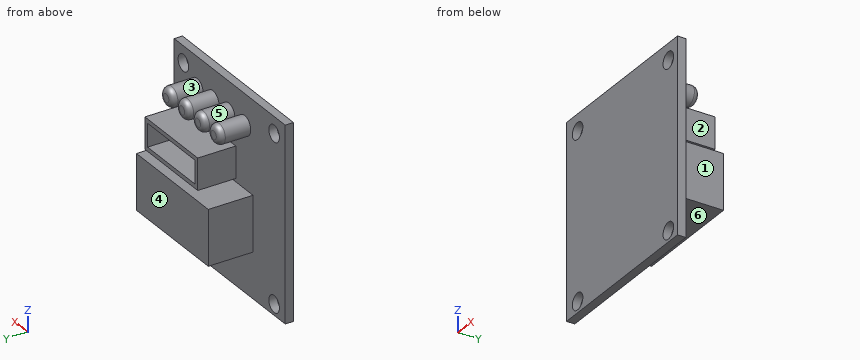
Autodesk Inventor part; units mm, degrees
ref_plane "YZ Plane" through (0, 0, 0) normal (1, 0, 0) x (0, 1, 0)
ref_plane "XZ Plane" through (0, 0, 0) normal (0, 1, 0) x (-1, 0, 0)
ref_plane "XY Plane" through (0, 0, 0) normal (0, 0, 1) x (1, 0, 0)
sketch "Sketch1" plane through (0, 0, 0) normal (0, 1, 0) x (-1, 0, 0)
  line L0 (0, 0) -> (-31.55, 0)
  line L1 (-31.55, 0) -> (-31.55, -35)
  line L2 (-31.55, -35) -> (0, -35)
  line L3 (0, -35) -> (0, 0)
  circle A0 centre (-3.15, -33) radius 1.5
  circle A1 centre (-28.95, -33) radius 1.5
  circle A2 centre (-3.15, -3) radius 1.5
  circle A3 centre (-28.95, -3) radius 1.5
  dimension "d0" = 31.55
  dimension "d1" = 35
  dimension "d2" = 3
  dimension "d3" = 25.8
  dimension "d4" = 2.6
  dimension "d5" = 30
  dimension "d6" = 2
extrude "Extrusion1" add sketch "Sketch1" along normal blind 1.5
sketch "Sketch2" plane through (0, 1.5, 0) normal (0, 1, 0) x (1, 0, 0)
  line L0 (9.15, 26.76) -> (29.55, 26.76)
  line L1 (29.55, 26.76) -> (29.55, 16.76)
  line L2 (29.55, 16.76) -> (9.15, 16.76)
  line L3 (9.15, 16.76) -> (9.15, 26.76)
  line L4 (31.55, 35) -> (0, 35)
  line L5 (29.05, 16.16) -> (14.05, 16.16)
  line L6 (14.05, 16.16) -> (14.05, 10.45)
  line L7 (14.05, 10.45) -> (29.05, 10.45)
  line L8 (29.05, 10.45) -> (29.05, 16.16)
  line L9 (28.3, 11.2) -> (14.8, 11.2)
  line L10 (14.8, 11.2) -> (14.8, 15.41)
  line L11 (14.8, 15.41) -> (28.3, 15.41)
  line L12 (28.3, 15.41) -> (28.3, 11.2)
  line L13 (31.55, 0) -> (31.55, 35)
  circle A0 centre (11.55, 5.6) radius 1.75
  circle A1 centre (16.05, 5.6) radius 1.75
  circle A2 centre (20.55, 5.6) radius 1.75
  circle A3 centre (25.05, 5.6) radius 1.75
  line L14 (0, 0) -> (31.55, 0)
  dimension "d9" = 10
  dimension "d10" = 20.4
  dimension "d11" = 8.24
  dimension "d12" = 2
  dimension "d15" = 15
  dimension "d16" = 5.71
  dimension "d17" = 2.5
  dimension "d18" = 10.45
  dimension "d19" = 0.75
  dimension "d22" = 4.5
  dimension "d23" = 4.5
  dimension "d24" = 4.5
  dimension "d25" = 6.5
  dimension "d26" = 5.6
  dimension "d27" = 3.5
extrude "Extrusion2" add sketch "Sketch2" along normal blind 8.11 contours L0 L1 L2 L3
extrude "Extrusion3" add sketch "Sketch2" along normal blind 6.9 contours L8 L7 L6 L5
extrude "Extrusion4" add sketch "Sketch2" along normal blind 5.6 contours A0 | A1 | A2 | A3
fillet "Fillet1" radius 1 4 edges at (9.8, 7.1, -5.6) (14.3, 7.1, -5.6) (18.8, 7.1, -5.6) (23.3, 7.1, -5.6)
properties part number "STEPPER DRIVER"
Design review of the part built by this model. Coordinates are the model's own, in mm. Face numbers are marked on the shaded views. A direction names the side the tool comes from. Give positions to 0.01 mm unless a question says otherwise; leave off trailing zeros. Order: outer loops, then holes, each group sorted by start corner. A loop starts at its lowest first (then second) coordinate and runs counter-clockwise, first axis right, second up. Notation, with made-up numbers: (40.25, -5.5) - (64.25, -5.5) arc R35 cw to (64.25, 33.5) - close; hole circle Ø4 at (77.5, 13.5). An arc over 180 degrees is marked (long way). Use CSV: the item, a comma, the result in double quotes. Start each with the question number.
Q1. Machinability: for the marked faces 1, 2 and 3, which of the approach directions +Z, -Z, +X, -X, +Y, -Y give a long, thin tool a straight path to every point of the face, cutting with its end or side? Answer none if there is none.
Q2. Take a section at D-D (z = -13). State the section outline as (x, y) points.
Q3. For P1, Ø4, axis at x = 8, y = 5.5, coming from the +Z side; P2, Ø4.5, axis at y = 4, z = -14, coming from the +X side; P3, Ø4, axis at y = 7, z = -20.5, coming from the -X side, all flat-tipped, find the tip position at first contact; note any pin that passes through.
Q4. Take a section at C-C (x = 3.15). State the section outline as (y, z) points.
Q5. For line 1 (Z direction, x = 3.15, y = 0.65); line 2 (Z direction, x = 22, y = 7.75); line 3 (X direction, y = 2, z = -14), list the stretches that pass through material, from the lowest coordinate up.
Q6. Draft analysis for pull direction Z (two halves, no side actions). For the marked faces 4, 5 and 6, state which applies: pulls with the +Z half, pulls with the -Z half, needs draft (parallel to the pull), parting line crosses it, or undercut.
Q7. Take a section at A-A (y = 4.25). State the section outline as (x, z) points, and give its area (3 significant figures).
Q8. Take a section at B-B (z = -3). State the section outline as (x, y) points, and give its area (3 significant figures).
Calculated:
1,face 1,"+Z, -Z, +X, +Y"
1,face 2,"+Z, +X, +Y"
1,face 3,"+Y"
2,outline,"(0, 0) - (31.55, 0) - (31.55, 1.5) - (29.05, 1.5) - (29.05, 8.4) - (28.3, 8.4) - (28.3, 1.5) - (14.8, 1.5) - (14.8, 8.4) - (14.05, 8.4) - (14.05, 1.5) - (0, 1.5) - close"
3,P1,"stops at z = -4.79"
3,P2,"stops at x = 29.05"
3,P3,"stops at x = 9.15"
4,outline,"(0, -35) - (1.5, -35) - (1.5, -34.5) - (0, -34.5) - close; (0, -31.5) - (1.5, -31.5) - (1.5, -4.5) - (0, -4.5) - close; (0, -1.5) - (1.5, -1.5) - (1.5, 0) - (0, 0) - close"
5,line 1,"z = -35 to -34.5, -31.5 to -4.5, -1.5 to 0"
5,line 2,"z = -26.76 to -16.76, -16.16 to -15.41, -11.2 to -10.45"
5,line 3,"x = 14.05 to 14.8, 28.3 to 29.05"
6,face 4,"needs draft"
6,face 5,"undercut"
6,face 6,"pulls with the -Z half"
7,outline,"(9.15, -26.76) - (29.55, -26.76) - (29.55, -16.76) - (9.15, -16.76) - close; circle Ø3.5 at (11.55, -5.6); (14.05, -16.16) - (29.05, -16.16) - (29.05, -10.45) - (14.05, -10.45) - close; circle Ø3.5 at (16.05, -5.6); circle Ø3.5 at (20.55, -5.6); circle Ø3.5 at (25.05, -5.6); hole (14.8, -15.41) - (28.3, -15.41) - (28.3, -11.2) - (14.8, -11.2) - close"
7,area,"271 mm²"
8,outline,"(0, 0) - (1.65, 0) - (1.65, 1.5) - (0, 1.5) - close; (4.65, 0) - (27.45, 0) - (27.45, 1.5) - (4.65, 1.5) - close; (30.45, 0) - (31.55, 0) - (31.55, 1.5) - (30.45, 1.5) - close"
8,area,"38.3 mm²"
